Autodesk Inventor part; units mm, degrees
ref_plane "XZ Plane" through (0, 0, 0) normal (0, 1, 0) x (-1, 0, 0)
ref_plane "XY Plane" through (0, 0, 0) normal (0, 0, 1) x (1, 0, 0)
sketch "スケッチ1" plane through (0, 0, 0) normal (0, 0, 1) x (1, 0, 0)
  circle A0 centre (-25.4, 0) radius 0.8
  point P0 (0, 0)
  dimension "d0" = 1.6
  dimension "d3" = 25.4
sketch "スケッチ2" plane through (0, 0, 0) normal (0, 1, 0) x (-1, 0, 0)
  line L0 (25.4, 0) -> (25.4, -9.625)
  line L1 (22.225, -12.8) -> (-22.225, -12.8)
  line L2 (-25.4, -9.625) -> (-25.4, 0)
  arc A0 (22.225, -12.8) -> (25.4, -9.625) centre (22.225, -9.625) ccw
  arc A1 (-25.4, -9.625) -> (-22.225, -12.8) centre (-22.225, -9.625) ccw
  point P0 (0, 0)
  point P1 (0, -12.8)
  dimension "d1" = 3.175
  dimension "d2" = 12.8
sweep "スイープ1" add profiles "スケッチ1" path "スケッチ2"
properties part number "stabbar_u5"
Read the model definition and answer for the solid it produces. Units are mm, in the model's axes. A direction names the side the tool comes from. Coordinates: 2 decimals unless noted, no trailing zeros. Order: outer loops, then holes, each group sorted by start corner. A loop starts at its lowest first (then second) coordinate and runs counter-clockwise, first axis right, second up. Notation, with made-up numbers: (65, -32) - (111, -32) arc R13 cw to (111, -11) - close; hole circle Ø11 at (81.25, 70). An arc over 180 degrees is marked (long way). Answer as a JSON object with one key per item and string values. Group by question number.
Item 1: A flat-ended cylindrical pin translates along its axis: P1, Ø8, axis at x = -20.5, z = -9.5, coming from the -Y side. Find the tip coordinate at first contact, or state that the pin passes through.
Item 2: A tool of negligible diameter and unlimited length cuts with its end or side. For faces 4 (the face through (-26.2, 0, -4.9)), 5 (the face through (-25, 0, 0)), from which of +Z, -Z, +X, -X, +Y, -Y can it reach the whole face along a straight path? Write none if from no direction.
Item 3: Section B-B (z = -5.25) is taken. Give the vertices of the cut face in (x, y), plus the area to 3 significant figures.
Item 4: The mould has two halves that part along X. Classify faces 1 (the face through (25, 0, 0)), 2 (the face through (26.2, 0, -4.7)), 3 (the face through (0, 0, -12)): +X half, -X half, draft (parallel to the pull), parting line (faces both ways), or undercut.
Item 5: Section A-A (y = 0) is taken. Give the vertices of the cut face in (x, z) (3 decimals).
Item 6: Consider probe 1 along X at (y, z) = (0, -9.75); probe 2 along X at (y, z) = (-0.3, -7); probe 3 along Z at (x, y) = (-0.5, 0.55). Determine where each line is inside the solid, lowest interval first. Write a range as from..to.
Item 7: Section C-C (x = 17) is taken. Give the vertices of the cut face in (y, z).
Results are:
{
 "1": {"P1": "stops at y = -0.8"},
 "2": {"face 4": "+Z", "face 5": "+Z, +X, -X, +Y, -Y"},
 "3": {"outline": "circle Ø1.6 at (-25.4, 0); circle Ø1.6 at (25.4, 0)", "area": "4.02 mm^2"},
 "4": {"face 1": "draft", "face 2": "undercut", "face 3": "undercut"},
 "5": {"outline": "(-26.2, -9.625) arc R3.975 ccw to (-22.225, -13.6) - (22.225, -13.6) arc R3.975 ccw to (26.2, -9.625) - (26.2, 0) - (24.6, 0) - (24.6, -9.625) arc R2.375 cw to (22.225, -12) - (-22.225, -12) arc R2.375 cw to (-24.6, -9.625) - (-24.6, 0) - (-26.2, 0) - close"},
 "6": {"probe 1": "x = -26.2..-24.6, 24.6..26.2", "probe 2": "x = -26.14..-24.66, 24.66..26.14", "probe 3": "z = -13.38..-12.22"},
 "7": {"outline": "circle Ø1.6 at (0, -12.8)"}
}
